Here's how the part is built. I have some questions about the finished solid (model axes, mm). A direction names the side the tool comes from. Coordinates: 2 decimals unless noted, no trailing zeros. Order: outer loops, then holes, each group sorted by start corner. A loop starts at its lowest first (then second) coordinate and runs counter-clockwise, first axis right, second up. Notation, with made-up numbers: (67, 3) - (83, 3) arc R30 ccw to (83, 40) - close; hole circle Ø7 at (0.25, -5.75). An arc over 180 degrees is marked (long way). Answer in a Markdown table with one row per item. Add a question column.
Item 1: I want a section at B-B (x = -14). Please give me the cut outline in (y, z) (3 decimals).
Item 2: If I drill on line 1 along X through (y, z) = (111.5, 3.5) (3 decimals); line 2 along Y through (x, z) = (-121, 4.5); line 3 along X through (y, z) = (-218.5, 2) (3 decimals), over which ranges is the centre line in solid material (lowest first)? Write a range as from..to.
Item 3: On a 3-axis mill with a long thin cutter (end or side, diameter ignored), from which of +Z, -Z, +X, -X, +Y, -Y can I reach the whole of each face in a straight line? I mean faces 5 (the flat face through (-4, -254, 9)), 6 (the flat face through (2, 146.05, 8)), 7 (the cylindrical face through (-148.58, 148.78, 17.48)). Say none if no direction works.
Item 4: I want a section at C-C (y = 173). Please give me the cut outline in (x, z) (3 decimals), plus the area to 3 significant figures.
Item 5: Thinking about a two-plate mould opening in Y: for faces 1 (the flat face through (-2, -146.05, 8)), 2 (the flat face through (304.8, -4, 9)), 3 (the flat face through (-4, 254, 9)), 4 (the cylindrical face through (148.58, -148.78, 17.48)), which applies, +Y half, -Y half, draft (parallel to the pull), parting line (faces both ways), or undercut?
Item 6: I want a section at D-D (x = -225.5). Please give me the cut outline in (y, z).
Item 7: I want a section at A-A (y = 91). Please give me the cut outline in (x, z) (3 decimals).
```python
from build123d import *

# Parameters (mm, degrees)
F0_W     = 609.6
F0_H     = 508
F1_DEPTH = 19.05
F3_DEPTH = 3.175
F5_DEPTH = 19.05
F6_W     = 438.15
F6_H     = 19.05
F7_DEPTH = 6.35


# Not quite as in the source:
# - a length typed as a fraction of an inch, garbled in the dataset ("3 / 203.2 mm" for 3/8 in), is restored


with BuildPart() as f1:
    # F0 (on Top) → F1 (new body)
    with BuildSketch(Plane.XY):
        Rectangle(F0_W, F0_H)
    extrude(amount=F1_DEPTH)

    # F2 (on face) → F3 (cut)
    with BuildSketch(Plane.XY.offset(19.05)):
        with BuildLine():
            ThreePointArc((152.4, 139.7), (148.6802561211, 148.6802561211), (139.7, 152.4))
            Line((139.7, 152.4), (-139.7, 152.4))
            ThreePointArc((-139.7, 152.4), (-148.6802561211, 148.6802561211), (-152.4, 139.7))
            Line((-152.4, 139.7), (-152.4, -139.7))
            ThreePointArc((-152.4, -139.7), (-148.6802561211, -148.6802561211), (-139.7, -152.4))
            Line((-139.7, -152.4), (139.7, -152.4))
            ThreePointArc((139.7, -152.4), (148.6802561211, -148.6802561211), (152.4, -139.7))
            Line((152.4, -139.7), (152.4, 139.7))
        make_face()
    extrude(amount=-F3_DEPTH, mode=Mode.SUBTRACT)

    # F4 (on face) → F5 (cut)
    with BuildSketch(Plane.XY.offset(15.875)):
        with BuildLine():
            ThreePointArc((146.05, 133.35), (142.3302561211, 142.3302561211), (133.35, 146.05))
            Line((133.35, 146.05), (-133.35, 146.05))
            ThreePointArc((-133.35, 146.05), (-142.3302561211, 142.3302561211), (-146.05, 133.35))
            Line((-146.05, 133.35), (-146.05, -133.35))
            ThreePointArc((-146.05, -133.35), (-142.3302561211, -142.3302561211), (-133.35, -146.05))
            Line((-133.35, -146.05), (133.35, -146.05))
            ThreePointArc((133.35, -146.05), (142.3302561211, -142.3302561211), (146.05, -133.35))
            Line((146.05, -133.35), (146.05, 133.35))
        make_face()
    extrude(amount=-F5_DEPTH, mode=Mode.SUBTRACT)

    # F6 (on face) → F7 (cut)
    with BuildSketch(Plane(origin=(0, 0, 0), x_dir=(1, 0, 0), z_dir=(0, 0, -1))):
        Polygon((-219.075, 228.6), (-238.125, 228.6), (-238.125, -228.6), (-219.075, -228.6), (-219.075, -209.55), align=None)
        with Locations((0, -219.075)):
            Rectangle(F6_W, F6_H)
        Polygon((219.075, 228.6), (219.075, -209.55), (219.075, -228.6), (238.125, -228.6), (238.125, 228.6), align=None)
    extrude(amount=-F7_DEPTH, mode=Mode.SUBTRACT)


solid = f1.part
```
Values follow:
| question | item | result |
|---|---|---|
| 1 | outline | (-254, 0) - (-146.05, 0) - (-146.05, 15.875) - (-152.4, 15.875) - (-152.4, 19.05) - (-254, 19.05) - close; (146.05, 0) - (209.55, 0) - (209.55, 6.35) - (228.6, 6.35) - (228.6, 0) - (254, 0) - (254, 19.05) - (152.4, 19.05) - (152.4, 15.875) - (146.05, 15.875) - close |
| 2 | line 1 | x = -304.8..-238.125, -219.075..-146.05, 146.05..219.075, 238.125..304.8 |
| 2 | line 2 | y = -254..-146.05, 146.05..209.55, 228.6..254 |
| 2 | line 3 | x = -304.8..-238.125, -219.075..219.075, 238.125..304.8 |
| 3 | face 5 | +Z, -Z, +X, -X, -Y |
| 3 | face 6 | +Z, -Z |
| 3 | face 7 | +Z |
| 4 | outline | (-304.8, 0) - (-238.125, 0) - (-238.125, 6.35) - (-219.075, 6.35) - (-219.075, 0) - (219.075, 0) - (219.075, 6.35) - (238.125, 6.35) - (238.125, 0) - (304.8, 0) - (304.8, 19.05) - (-304.8, 19.05) - close |
| 4 | area | 11,400 mm^2 |
| 5 | face 1 | undercut |
| 5 | face 2 | draft |
| 5 | face 3 | +Y half |
| 5 | face 4 | undercut |
| 6 | outline | (-254, 0) - (-228.6, 0) - (-228.6, 6.35) - (228.6, 6.35) - (228.6, 0) - (254, 0) - (254, 19.05) - (-254, 19.05) - close |
| 7 | outline | (-304.8, 0) - (-238.125, 0) - (-238.125, 6.35) - (-219.075, 6.35) - (-219.075, 0) - (-146.05, 0) - (-146.05, 15.875) - (-152.4, 15.875) - (-152.4, 19.05) - (-304.8, 19.05) - close; (146.05, 0) - (219.075, 0) - (219.075, 6.35) - (238.125, 6.35) - (238.125, 0) - (304.8, 0) - (304.8, 19.05) - (152.4, 19.05) - (152.4, 15.875) - (146.05, 15.875) - close |
